from build123d import *

# Parameters (mm, degrees)
SKETCH_W   = 200
SKETCH_H   = 130
SKETCH_R   = 40
SKETCH_R_2 = 1.5625
PAD_DEPTH  = 12
FILLET_R   = 3


with BuildPart() as part:
    # Sketch → Pad (new body)
    with BuildSketch(Plane.XY):
        with Locations((100, 65)):
            Rectangle(SKETCH_W, SKETCH_H)
        with Locations((100, 65)):
            Circle(SKETCH_R, mode=Mode.SUBTRACT)
        with Locations((45, 115)):
            Circle(SKETCH_R_2, mode=Mode.SUBTRACT)
        with Locations((45, 15)):
            Circle(SKETCH_R_2, mode=Mode.SUBTRACT)
        with Locations((155, 115)):
            Circle(SKETCH_R_2, mode=Mode.SUBTRACT)
        with Locations((155, 15)):
            Circle(SKETCH_R_2, mode=Mode.SUBTRACT)
        with Locations((185, 30)):
            Circle(SKETCH_R_2, mode=Mode.SUBTRACT)
        with Locations((135.355339, 100.355339)):
            Circle(SKETCH_R_2, mode=Mode.SUBTRACT)
        with Locations((64.644661, 29.644661)):
            Circle(SKETCH_R_2, mode=Mode.SUBTRACT)
        with Locations((64.644661, 100.355339)):
            Circle(SKETCH_R_2, mode=Mode.SUBTRACT)
        with Locations((135.355339, 29.644661)):
            Circle(SKETCH_R_2, mode=Mode.SUBTRACT)
        with Locations((175, 20)):
            Circle(SKETCH_R_2, mode=Mode.SUBTRACT)
        with Locations((175, 40)):
            Circle(SKETCH_R_2, mode=Mode.SUBTRACT)
        with Locations((185, 50)):
            Circle(SKETCH_R_2, mode=Mode.SUBTRACT)
        with Locations((175, 90)):
            Circle(SKETCH_R_2, mode=Mode.SUBTRACT)
        with Locations((175, 110)):
            Circle(SKETCH_R_2, mode=Mode.SUBTRACT)
        with Locations((185, 80)):
            Circle(SKETCH_R_2, mode=Mode.SUBTRACT)
        with Locations((185, 100)):
            Circle(SKETCH_R_2, mode=Mode.SUBTRACT)
        with Locations((15, 30)):
            Circle(SKETCH_R_2, mode=Mode.SUBTRACT)
        with Locations((25, 20)):
            Circle(SKETCH_R_2, mode=Mode.SUBTRACT)
        with Locations((25, 40)):
            Circle(SKETCH_R_2, mode=Mode.SUBTRACT)
        with Locations((15, 50)):
            Circle(SKETCH_R_2, mode=Mode.SUBTRACT)
        with Locations((25, 90)):
            Circle(SKETCH_R_2, mode=Mode.SUBTRACT)
        with Locations((25, 110)):
            Circle(SKETCH_R_2, mode=Mode.SUBTRACT)
        with Locations((15, 80)):
            Circle(SKETCH_R_2, mode=Mode.SUBTRACT)
        with Locations((15, 100)):
            Circle(SKETCH_R_2, mode=Mode.SUBTRACT)
        with Locations((15, 120)):
            Circle(SKETCH_R_2, mode=Mode.SUBTRACT)
        with Locations((185, 120)):
            Circle(SKETCH_R_2, mode=Mode.SUBTRACT)
    extrude(amount=PAD_DEPTH)

    # Fillet
    fillet_edges = [part.edges().sort_by_distance(p)[0] for p in [
        (200, 130, 6),
        (0, 130, 6),
        (200, 0, 6),
        (0, 0, 6),
    ]]
    fillet(fillet_edges, radius=FILLET_R)


solid = part.part
Can you work these out from the model? Positions are in its coordinate system, mm. Round coordinates to 2 decimals unless told otherwise and drop trailing zeros. Write each loop counter-clockwise with the first axis right and the second up, starting at its lowest first coordinate (ties: lowest second). Pieces come first, ordered by that corner, then holes. Notation, with made-up numbers: (-34.75, 29.25) -> (3.25, 29.25) arc R6 ccw to (3.25, 33.25) -> close; hole circle Ø6 at (16, -22). An arc over 180 degrees is marked (long way). One line per question, with ' | ' between items. Start each with the question number.
1) Suppose I cut it at B-B on z = 6.75. Count the separate pieces of the cut face and the enclosed holes in it, then the cut area to 3 significant figures.
2) I need wall thicknesses on line 1 (Y direction, x = 155, z = 9); line 2 (Y direction, x = 185, z = 7.75); line 3 (X direction, y = 115, z = 4). Which ranges of each line are inside material? Lowest first, please. Write a range as [from, to].
3) I'm going to push a flat-ended pin straight in: P1, Ø2.5, axis at x = 15, y = 80, coming from the -Z side. Where does the tip first touch, or does it pass through?
4) Suppose I cut it at A-A on x = 121. Write out the boundary of the cut face in (y, z).
5) If we mould it in two halves opening along X, with no side actions, what happens to faces 1 (the cylindrical face through (138.153, 77.015, 5.916)), 2 (the flat face through (99, 109, 0)), 3 (the flat face through (200, 64, 6))? For each: released by +X, released by -X, zero draft, split by the parting line, or undercut.
Return value:
1) separate pieces: 1 | enclosed holes: 27 | area: 20,800 mm2
2) line 1: y = [0, 13.44], [16.56, 113.44], [116.56, 130] | line 2: y = [0, 28.44], [31.56, 48.44], [51.56, 78.44], [81.56, 98.44], [101.56, 118.44], [121.56, 130] | line 3: x = [0, 43.44], [46.56, 153.44], [156.56, 200]
3) P1: passes through
4) outline: (0, 0) -> (30.96, 0) -> (30.96, 12) -> (0, 12) -> close; (99.04, 0) -> (130, 0) -> (130, 12) -> (99.04, 12) -> close
5) face 1: undercut | face 2: zero draft | face 3: released by +X
